from build123d import *

# Parameters (mm, degrees)
BOSS_EXTRUDE1_DEPTH                               = 3.175
SKETCH2_R                                         = 2.413
SKETCH2_R_2                                       = 0.79375
CUT_EXTRUDE1_DEPTH                                = 60.989858518
CSK_FOR_4_FLAT_HEAD_MACHINE_SCREW_100_D           = 3.2639
CSK_FOR_4_FLAT_HEAD_MACHINE_SCREW_100_CSINK_D     = 5.715
CSK_FOR_4_FLAT_HEAD_MACHINE_SCREW_100_CSINK_ANGLE = 100
SKETCH5_R                                         = 2.38125
SKETCH5_R_2                                       = 0.396875
CUT_EXTRUDE2_DEPTH                                = 60.989858518
BOSS_EXTRUDE2_DEPTH                               = 3.175


with BuildPart() as part:
    # Sketch1 → Boss-Extrude1 (new body)
    with BuildSketch(Plane(origin=(0, 0, 0), x_dir=(1, 0, 0), z_dir=(0, 1, 0))):
        with BuildLine():
            Line((0, 31.75), (-50.8, 31.75))
            Line((-50.8, 31.75), (-50.8, -31.75))
            Line((-50.8, -31.75), (0, -31.75))
            ThreePointArc((0, -31.75), (31.75, 0), (0, 31.75))
        make_face()
    extrude(amount=BOSS_EXTRUDE1_DEPTH)

    # Sketch2 → Cut-Extrude1 (cut, through all)
    with BuildSketch(Plane(origin=(0, 3.175, 0), x_dir=(1, 0, 0), z_dir=(0, 1, 0))):
        with Locations(Location((0, 0, 0), (0, 0, 270))):
            Circle(SKETCH2_R)
        with Locations(Location((-19.165786135, -5.680153436, 0), (0, 0, 270))):
            Circle(SKETCH2_R_2)
        with Locations(Location((-4.607724074, 12.589841237, 0), (0, 0, 270))):
            Circle(SKETCH2_R_2)
        with Locations(Location((3.935524409, -9.152807674, 0), (0, 0, 270))):
            Circle(SKETCH2_R_2)
    extrude(amount=-CUT_EXTRUDE1_DEPTH, mode=Mode.SUBTRACT)

    # CSK for #4 Flat Head Machine Screw (100)1 (through all)
    with Locations(Plane(origin=(0, 3.175, 0), x_dir=(1, 0, 0), z_dir=(0, 1, 0))):
        with Locations((3.935524409, -9.152807674), (-19.165786135, -5.680153436), (-4.607724074, 12.589841237)):
            CounterSinkHole(CSK_FOR_4_FLAT_HEAD_MACHINE_SCREW_100_D / 2, CSK_FOR_4_FLAT_HEAD_MACHINE_SCREW_100_CSINK_D / 2, counter_sink_angle=CSK_FOR_4_FLAT_HEAD_MACHINE_SCREW_100_CSINK_ANGLE)

    # Sketch5 → Cut-Extrude2 (cut, through all)
    with BuildSketch(Plane(origin=(0, 3.175, 0), x_dir=(1, 0, 0), z_dir=(0, 1, 0))):
        with Locations(Location((15.24, 21.59, 0), (0, 0, 270))):
            Circle(SKETCH5_R)
        with Locations(Location((-41.91, 30.48, 0), (0, 0, 270))):
            Circle(SKETCH5_R_2)
    extrude(amount=-CUT_EXTRUDE2_DEPTH, mode=Mode.SUBTRACT)

    # Sketch6 → Boss-Extrude2 (add)
    with BuildSketch(Plane(origin=(0, 0, -31.75), x_dir=(-1, 0, 0), z_dir=(0, 0, -1))):
        with BuildLine():
            Line((50.8, 3.175), (19.05, 3.175))
            Line((19.05, 3.175), (19.05, -28.575))
            Line((19.05, -28.575), (22.799338861, -28.575))
            ThreePointArc((22.799338861, -28.575), (32.546509941, -10.119826243), (50.8, 0))
            Line((50.8, 0), (50.8, 3.175))
        make_face()
    boss_extrude2 = extrude(amount=BOSS_EXTRUDE2_DEPTH)

    # Mirror1: Boss-Extrude2 across plane
    add(boss_extrude2.mirror(Plane.XY))


solid = part.part
Work out the finished part from the listing and answer in its coordinate system (mm). A direction names the side the tool comes from. Coordinates: 2 decimals unless noted, no trailing zeros. Order: outer loops, then holes, each group sorted by start corner. A loop starts at its lowest first (then second) coordinate and runs counter-clockwise, first axis right, second up. Notation, with made-up numbers: (17, 19) - (35, 19) arc R22 cw to (35, 51) - close; hole circle Ø10 at (54, 21.5). An arc over 180 degrees is marked (long way). Put each result on its own line as item: value. Start each with the question number.
1) For faces 4 (the flat face through (-28, -11, 31.75)), 5 (the flat face through (-10, 2, 31.75)), 6 (the flat face through (-9, 2, -31.75)), determine the directions among +Z, -Z, +X, -X, +Y, -Y from which every point of the face is accessible in a straight line to the end or side of a thin tool.
2) Find section B-B (y = -26). Give the vertices of the cut face in (x, z) (3 decimals).
3) Find the intervals of material crossed by line 1 (Z direction, x = -29, y = -2.5) (3 decimals); line 2 (Y direction, x = -41.5, z = -0.5) (3 decimals), in increasing order. Write a range as from..to.
4) Find section D-D (z = 15). Give the vertices of the cut face in (x, y) (3 decimals), plus the area to 3 significant figures.
5) For a pull along X with two mould halves and no side action, classify faces 1 (the flat face through (-10, 0, 0)), 2 (the flat face through (-50.8, 2, 0)), 3 (the cylindrical face through (-4.254, 1.058, -10.997)) as released by +X, released by -X, zero draft, split by the parting line, or undercut.
6) Find section A-A (z = 0). Give the vertices of the cut face in (x, y) (3 decimals), plus the area to 3 significant figures.
7) Flat-ended cylindrical pins translate along their axes: pin 1 (3.5 mm diameter, centred on x = -11.5, y = 1, fed in from +Z); pin 2 (1.5 mm diameter, centred on x = -34, z = -26, fed in from -Y); pin 3 (1 mm diameter, centred on y = -19.5, z = -34, fed in from +X). Find the tip coordinate at first contact, or state that the pin passes through.
8) Find section C-C (x = -44.5). Give the vertices of the cut face in (y, z) (3 decimals), plus the area to 3 significant figures.
Results list:
1. face 4: +X, -X, -Y
1. face 5: +Z, +X, +Y, -Y
1. face 6: -Z, +X, +Y, -Y
2. outline: (-23.41, -34.925) - (-19.05, -34.925) - (-19.05, -31.75) - (-23.41, -31.75) - close; (-23.41, 31.75) - (-19.05, 31.75) - (-19.05, 34.925) - (-23.41, 34.925) - close
3. line 1: z = -34.925..-31.75, 31.75..34.925
3. line 2: y = 0..3.175
4. outline: (-50.8, 0) - (27.983, 0) - (27.983, 3.175) - (-50.8, 3.175) - close
4. area: 250 mm^2
5. face 1: zero draft
5. face 2: released by -X
5. face 3: undercut
6. outline: (-50.8, 0) - (-2.413, 0) - (-2.413, 3.175) - (-50.8, 3.175) - close; (2.413, 0) - (31.75, 0) - (31.75, 3.175) - (2.413, 3.175) - close
6. area: 247 mm^2
7. pin 1: stops at z = 31.75
7. pin 2: stops at y = 0
7. pin 3: stops at x = -19.05
8. outline: (-2, -34.925) - (3.175, -34.925) - (3.175, 34.925) - (-2, 34.925) - (-2, 31.75) - (0, 31.75) - (0, -31.75) - (-2, -31.75) - close
8. area: 234 mm^2
